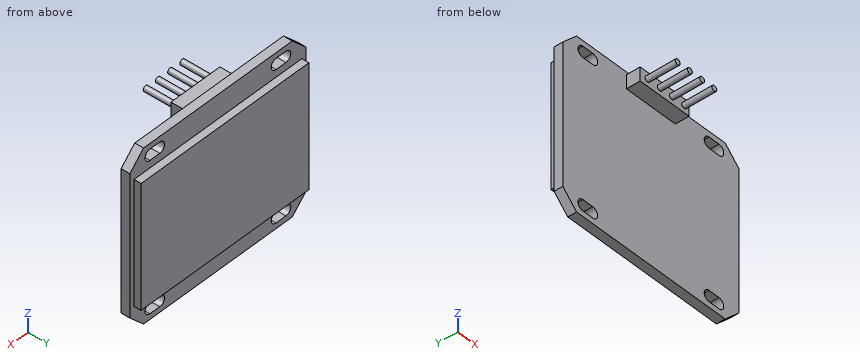
from build123d import *

# Parameters (mm, degrees)
SKETCH_1_W             = 36
SKETCH_1_H             = 31.2
EXTRUDE_1_DEPTH        = 1.6
SKETCH_2_W             = 34.3
SKETCH_2_H             = 22.5
EXTRUDE_2_DEPTH        = 1.3
CUT_EXTRUDE_1_DEPTH    = 24.872997298
CHAMFER_1_SIZE         = 2.8
SKETCH_4_W             = 10
SKETCH_4_H             = 2.5
EXTRUDE_3_DEPTH        = 2.5
SKETCH_5_R             = 0.5
EXTRUDE_4_DEPTH        = 5.5
PATTERN_LINEAR_1_COUNT = 4
PATTERN_LINEAR_1_PITCH = 2.5


with BuildPart() as part:
    # 草图1 → 凸台-拉伸1 (new body)
    with BuildSketch(Plane(origin=(0, 0, 0), x_dir=(1, 0, 0), z_dir=(0, 1, 0))):
        Rectangle(SKETCH_1_W, SKETCH_1_H)
    extrude(amount=EXTRUDE_1_DEPTH)

    # 草图2 → 凸台-拉伸2 (add)
    with BuildSketch(Plane(origin=(0, 1.6, 0), x_dir=(1, 0, 0), z_dir=(0, 1, 0))):
        Rectangle(SKETCH_2_W, SKETCH_2_H)
    extrude(amount=EXTRUDE_2_DEPTH)

    # 草图3 → 切除-拉伸1 (cut, through all)
    with BuildSketch(Plane(origin=(0, 1.6, 0), x_dir=(1, 0, 0), z_dir=(0, 1, 0))):
        with BuildLine():
            Line((-13.9, 14.6), (-11.9, 14.6))
            ThreePointArc((-11.9, 14.6), (-10.9, 13.6), (-11.9, 12.6))
            Line((-11.9, 12.6), (-13.9, 12.6))
            ThreePointArc((-13.9, 12.6), (-14.9, 13.6), (-13.9, 14.6))
        make_face()
        with BuildLine():
            Line((13.9, 14.6), (11.9, 14.6))
            ThreePointArc((11.9, 14.6), (10.9, 13.6), (11.9, 12.6))
            Line((11.9, 12.6), (13.9, 12.6))
            ThreePointArc((13.9, 12.6), (14.9, 13.6), (13.9, 14.6))
        make_face()
        with BuildLine():
            Line((13.9, -14.6), (11.9, -14.6))
            ThreePointArc((11.9, -14.6), (10.9, -13.6), (11.9, -12.6))
            Line((11.9, -12.6), (13.9, -12.6))
            ThreePointArc((13.9, -12.6), (14.9, -13.6), (13.9, -14.6))
        make_face()
        with BuildLine():
            Line((-13.9, -14.6), (-11.9, -14.6))
            ThreePointArc((-11.9, -14.6), (-10.9, -13.6), (-11.9, -12.6))
            Line((-11.9, -12.6), (-13.9, -12.6))
            ThreePointArc((-13.9, -12.6), (-14.9, -13.6), (-13.9, -14.6))
        make_face()
    extrude(amount=-CUT_EXTRUDE_1_DEPTH, mode=Mode.SUBTRACT)

    # 倒角1
    chamfer_1_edges = [part.edges().sort_by_distance(p)[0] for p in [
        (18, 0.8, 15.6),
        (-18, 0.8, 15.6),
        (-18, 0.8, -15.6),
        (18, 0.8, -15.6),
    ]]
    chamfer(chamfer_1_edges, length=CHAMFER_1_SIZE)

    # 草图4 → 凸台-拉伸3 (add)
    with BuildSketch(Plane.XZ):
        with Locations((0, 13.85)):
            Rectangle(SKETCH_4_W, SKETCH_4_H)
    extrude(amount=EXTRUDE_3_DEPTH)

    # 草图5 → 凸台-拉伸4 (add)
    with BuildSketch(Plane.XZ.offset(2.5)):
        with Locations(Location((-3.5, 13.85, 0), (0, 0, 90))):
            Circle(SKETCH_5_R)
    extrude_4 = extrude(amount=EXTRUDE_4_DEPTH)

    # 阵列(线性)1: 凸台-拉伸4 ×4
    with Locations(*[(i * PATTERN_LINEAR_1_PITCH, 0, 0) for i in range(1, PATTERN_LINEAR_1_COUNT)]):
        add(extrude_4)


solid = part.part
The listing builds one solid part. Answer for the finished solid, in the listing's coordinates (mm). Give positions to 0.01 mm unless a question says otherwise; leave off trailing zeros. Order: outer loops, then holes, each group sorted by start corner. A loop starts at its lowest first (then second) coordinate and runs counter-clockwise, first axis right, second up. Notation, with made-up numbers: (-30.5, 56.25) - (-19.5, 56.25) arc R11 cw to (-19.5, 62.25) - close; hole circle Ø6 at (-22.5, 78). An arc over 180 degrees is marked (long way). Use one line per item in the form item = value.
1) Find section C-C on x = -3.5. Determine the outline of the cut face in (y, z), and give its area (3 significant figures).
Verdict:
outline = (-8, 13.35) - (-2.5, 13.35) - (-2.5, 12.6) - (0, 12.6) - (0, -15.6) - (1.6, -15.6) - (1.6, -11.25) - (2.9, -11.25) - (2.9, 11.25) - (1.6, 11.25) - (1.6, 15.6) - (0, 15.6) - (0, 15.1) - (-2.5, 15.1) - (-2.5, 14.35) - (-8, 14.35) - close
area = 90.9 mm^2
2) Consider probe 1 along X at (y, z) = (-6.5, 14); probe 2 along Y at (x, z) = (-9.5, 2); probe 3 along Z at (x, y) = (-4, -1.25). Determine where each line is inside the solid, lowest interval first. Write a range as [from, to].
Verdict:
probe_1 = [-3.98, -3.02], [-1.48, -0.52], [1.02, 1.98], [3.52, 4.48]
probe_2 = [0, 2.9]
probe_3 = [12.6, 15.1]
3) Find section D-D on z = 1. Determine the outline of the cut face in (x, y), and give its area (3 significant figures).
Verdict:
outline = (-18, 0) - (18, 0) - (18, 1.6) - (17.15, 1.6) - (17.15, 2.9) - (-17.15, 2.9) - (-17.15, 1.6) - (-18, 1.6) - close
area = 102 mm^2
4) Find section A-A on z = 13.85. Give the number of separate pieces and of enclosed holes in the cut face, and give its area (3 significant figures).
Verdict:
separate_pieces = 3
enclosed_holes = 0
area = 88.6 mm^2
5) Each of these flat-tipped pins is pushed along its axis until it touches: pin 1 (2 mm diameter, centred on y = -0.5, z = 14, fed in from -X); pin 2 (5 mm diameter, centred on x = 6, y = -3, fed in from +Z); pin 3 (2 mm diameter, centred on x = 3, y = -2, fed in from -Z); pin 4 (6 mm diameter, centred on y = -5, z = 5.5, fed in from +X). Where does it stop, or does it pass through?
Verdict:
pin_1 = -17.67
pin_2 = 15.1
pin_3 = 12.6
pin_4 = through
6) Find section B-B on y = -7. Determine the outline of the cut face in (x, z).
Verdict:
outline = circle Ø1 at (-3.5, 13.85); circle Ø1 at (-1, 13.85); circle Ø1 at (1.5, 13.85); circle Ø1 at (4, 13.85)
